Could you check a few things on this drawing? It's one solid part, dimensions in mm from its lowest x, y, z. Round coordinates to 2 decimals unless told otherwise and drop trailing zeros. Write each loop counter-clockwise with the first axis right and the second up, starting at its lowest first coordinate (ties: lowest second). Pieces come first, ordered by that corner, then holes. Notation, with made-up numbers: (-23, -8.5) -> (-5, -8.5) arc R18 cw to (-5, -0.5) -> close; hole circle Ø4 at (82.25, -3.75). An arc over 180 degrees is marked (long way). Answer as CSV lines item,"result".
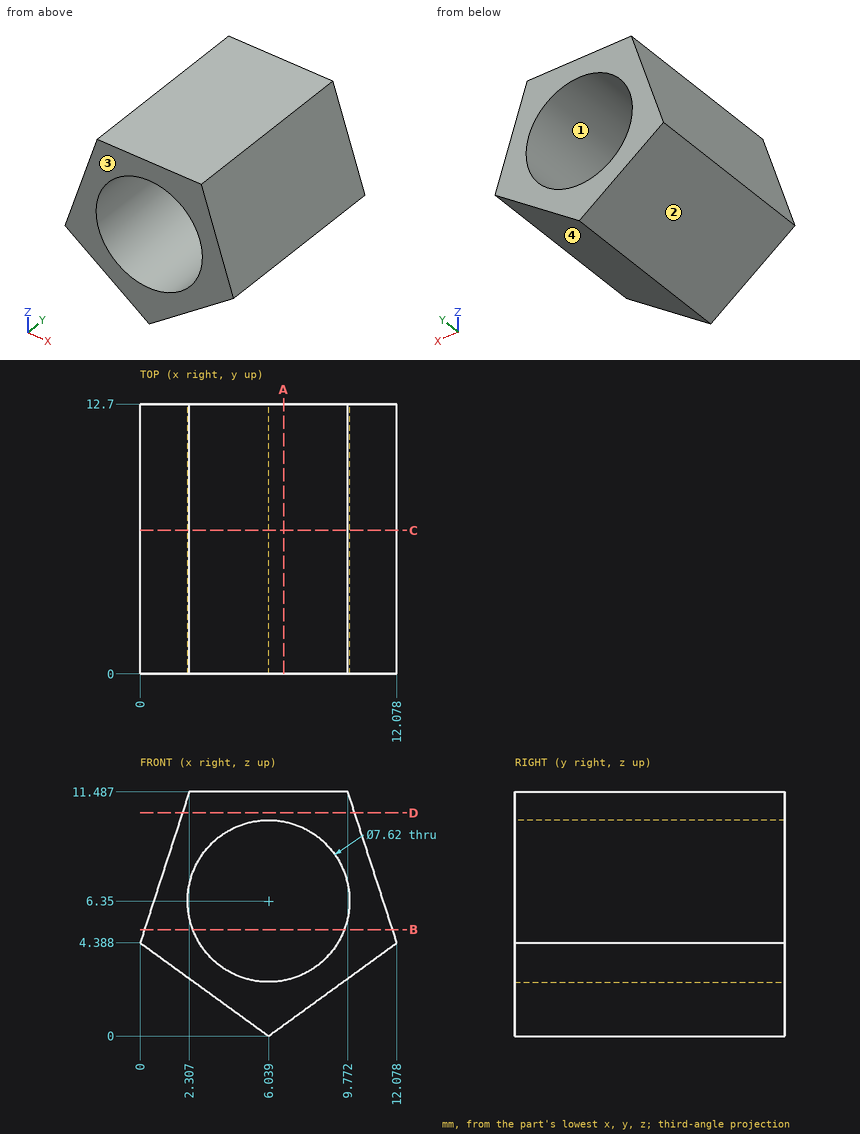
1. If we mould it in two halves opening along X, with no side actions, what happens to the marked faces 1, 2, 3 and 4? For each: released by +X, released by -X, zero draft, split by the parting line, or undercut.
Numbers:
face 1,"undercut"
face 2,"released by -X"
face 3,"zero draft"
face 4,"released by +X"
2. For pin 1 Ø5 at (y, z) = (7.5, 10) entering from +X; pin 2 Ø5 at (x, y) = (9, 2) entering from -Z (1 decimal), each with a flat end and sliding along its axis, tell me the tip position at first contact or that it passes through.
Numbers:
pin 1,"stops at x = 11.07"
pin 2,"stops at z = 0.3"
3. Suppose I cut it at D-D on z = 10.5. Please give me the cut outline in (x, y).
Numbers:
outline,"(1.99, 0) -> (10.09, 0) -> (10.09, 12.7) -> (1.99, 12.7) -> close"
4. If I drill on line 1 (X direction, y = 10.25, z = 6.35); line 2 (X direction, y = 11, z = 6.75); line 3 (Z direction, x = 7.5, y = 7.5), over which ranges is the centre line in solid material (lowest first)?
Numbers:
line 1,"x = 0.64 to 2.23, 9.85 to 11.44"
line 2,"x = 0.77 to 2.25, 9.83 to 11.31"
line 3,"z = 1.06 to 2.83, 9.87 to 11.49"
5. Suppose I cut it at C-C on y = 6.75. Please give me the cut outline in (x, z).
Numbers:
outline,"(0, 4.39) -> (6.04, 0) -> (12.08, 4.39) -> (9.77, 11.49) -> (2.31, 11.49) -> close; hole circle Ø7.62 at (6.04, 6.35)"
6. Suppose I cut it at B-B on z = 5. Please give me the cut outline in (x, y).
Numbers:
outline,"(0.2, 0) -> (2.48, 0) -> (2.48, 12.7) -> (0.2, 12.7) -> close; (9.6, 0) -> (11.88, 0) -> (11.88, 12.7) -> (9.6, 12.7) -> close"
7. Suppose I cut it at A-A on x = 6.75. Please give me the cut outline in (y, z).
Numbers:
outline,"(0, 0.52) -> (12.7, 0.52) -> (12.7, 2.61) -> (0, 2.61) -> close; (0, 10.09) -> (12.7, 10.09) -> (12.7, 11.49) -> (0, 11.49) -> close"
